Autodesk Inventor part; units mm, degrees
ref_plane "YZ Plane" through (0, 0, 0) normal (1, 0, 0) x (0, 1, 0)
ref_plane "XZ Plane" through (0, 0, 0) normal (0, 1, 0) x (-1, 0, 0)
ref_plane "XY Plane" through (0, 0, 0) normal (0, 0, 1) x (1, 0, 0)
sketch "スケッチ1" plane through (0, 0, 0) normal (0, 0, 1) x (1, 0, 0)
  circle A0 centre (0, 0) radius 1.5
  dimension "d0" = 3
extrude "押し出し1" add sketch "スケッチ1" along normal blind 6
sketch "スケッチ2" plane through (0, 0, 6) normal (0, 0, 1) x (1, 0, 0)
  circle A0 centre (0, 0) radius 1.5
  circle A1 centre (0, 0) radius 3
  dimension "d3" = 6
extrude "押し出し2" add sketch "スケッチ2" along normal blind 2 contours A0 | A1
fillet "フィレット1" radius 2 1 edges at (-3, 0, 8)
thread "ねじ1"
sketch "スケッチ3" plane through (0, 0, 0) normal (0, 0, -1) x (-1, 0, 0)
  circle A0 centre (0, 0) radius 1.5
extrude "押し出し3" add sketch "スケッチ3" along normal blind 9
sketch "スケッチ4" plane through (0, 0, -9) normal (0, 0, -1) x (-1, 0, 0)
  circle A0 centre (0, 0) radius 1.5
extrude "押し出し4" add sketch "スケッチ4" along normal blind 5
sketch "スケッチ5" plane through (0, 0, -14) normal (0, 0, -1) x (-1, 0, 0)
  circle A0 centre (0, 0) radius 1.5
  dimension "d13" = 3
extrude "押し出し5" add sketch "スケッチ5" along normal blind 5
properties part number "SB　25mmなべネジ" material "鋼、高強度、低合金"
Input: part model. Units: mm. Frame: model coordinates. A direction names the side the tool comes from. Coordinates: 2 decimals unless noted, no trailing zeros. Loops run counter-clockwise (first coordinate to the right, second up) from the corner with the lowest first, then second, coordinate; pieces in that order, holes last.
(1) Section A-A on z = -10. Return the cut outline in (x, y), then the cut area to 3 significant figures.
(2) Set-up query: faces 1 (the face through (1.3, -1.3, 6)), 2 (the face through (0, 0, -19)). Return all of +Z, -Z, +X, -X, +Y, -Y with unobstructed straight access to the full face (end or side cutting, diameter ignored); none if empty.
(3) Material intervals for probe 1 along Y at (x, z) = (0, -15.75); probe 2 along Y at (x, z) = (1.25, 2.75); probe 3 along Z at (x, y) = (-2.5, 0.5), sorted ascending.
(4) First-contact query: pin 1 Ø3 at (y, z) = (1.5, 1.5) entering from +X; pin 2 Ø1.5 at (y, z) = (-0.5, -10) entering from -X; pin 3 Ø1.5 at (x, y) = (0, 2) entering from +Z. Flat tips, straight axial feed; report the tip coordinate or a pass-through.
Data:
1. outline: circle Ø3 at (0, 0)
1. area: 7.07 mm2
2. face 1: -Z
2. face 2: -Z, +X, -X, +Y, -Y
3. probe 1: y = -1.5 to 1.5
3. probe 2: y = -0.83 to 0.83
3. probe 3: z = 6 to 7.26
4. pin 1: stops at x = 1.5
4. pin 2: stops at x = -1.5
4. pin 3: stops at z = 7.98
